The listing builds one solid part. Answer for the finished solid, in the listing's coordinates (mm). A direction names the side the tool comes from. Coordinates: 2 decimals unless noted, no trailing zeros. Order: outer loops, then holes, each group sorted by start corner. A loop starts at its lowest first (then second) coordinate and runs counter-clockwise, first axis right, second up. Notation, with made-up numbers: (-6, -21.5) -> (43, -21.5) arc R16 cw to (43, -14.5) -> close; hole circle Ø11 at (-35, 16). An arc over 180 degrees is marked (long way). Answer in a Markdown table with one row per item. Add a question column.
```python
from build123d import *

# Parameters (mm, degrees)
BOSS_EXTRUDE1_DEPTH     = 2
SKETCH2_W               = 3.5
SKETCH2_H               = 2
CUT_EXTRUDE1_DEPTH      = 22
BOSS_EXTRUDE2_DEPTH     = 7
BOSS_EXTRUDE3_DEPTH     = 6
SKETCH5_R               = 2.25
CUT_EXTRUDE3_DEPTH      = 37
CUT_EXTRUDE3_DEPTH_BACK = 37
FILLET1_R               = 3
FILLET2_R               = 0.5
CUT_EXTRUDE4_DEPTH      = 37
FILLET3_R               = 0.5
FILLET4_R               = 0.5
CUT_EXTRUDE5_DEPTH      = 10
FILLET8_R               = 1
SKETCH8_W               = 0.1
SKETCH8_H               = 1
CUT_EXTRUDE6_DEPTH      = 0.1
SKETCH11_R              = 50.237983701
CUT_EXTRUDE8_DEPTH      = 11
CUT_EXTRUDE8_DEPTH_BACK = 1


with BuildPart() as part:
    # Sketch1 → Boss-Extrude1 (new body)
    with BuildSketch(Plane(origin=(0, 0, 0), x_dir=(1, 0, 0), z_dir=(0, 1, 0))):
        with BuildLine():
            Line((-27.424590139, -24.837307739), (27.424590139, -24.837307739))
            ThreePointArc((27.424590139, -24.837307739), (37, 0), (27.424590139, 24.837307739))
            Line((27.424590139, 24.837307739), (-27.424590139, 24.837307739))
            ThreePointArc((-27.424590139, 24.837307739), (-37, 0), (-27.424590139, -24.837307739))
        make_face()
    extrude(amount=BOSS_EXTRUDE1_DEPTH)

    # Sketch2 → Cut-Extrude1 (cut)
    with BuildSketch(Plane.XZ):
        Polygon((-8, 0), (-8, 9.5), (-11, 9.5), (-11, -9.5), (-8, -9.5), align=None)
        with Locations((-9.75, 0)):
            Rectangle(SKETCH2_W, SKETCH2_H)
    extrude(amount=-CUT_EXTRUDE1_DEPTH, mode=Mode.SUBTRACT)

    # Sketch3 → Boss-Extrude2 (add)
    with BuildSketch(Plane(origin=(0, 2, 0), x_dir=(1, 0, 0), z_dir=(0, 1, 0))):
        Polygon((2.9, 11.6), (2.9, 10.1), (19, 10.1), (20.5, 10.1), (20.5, 11.6), align=None)
        Polygon((20.5, 10.1), (19, 10.1), (19, -10.1), (19, -11.6), (20.5, -11.6), align=None)
        Polygon((19, -11.6), (19, -10.1), (-14.6, -10.1), (-16.1, -10.1), (-16.1, -11.6), align=None)
        Polygon((-14.6, 10.1), (2.9, 10.1), (2.9, 11.6), (-16.1, 11.6), (-16.1, 10.1), align=None)
    extrude(amount=BOSS_EXTRUDE2_DEPTH)

    # Sketch4 → Boss-Extrude3 (add)
    with BuildSketch(Plane.XZ):
        Polygon((-8, 0), (-8.02303658, 9.318964787), (-3, 9.318964787), (-3, -9.5), (-8, -9.5), align=None)
    extrude(amount=BOSS_EXTRUDE3_DEPTH)

    # Sketch5 → Cut-Extrude3 (cut, two sides)
    with BuildSketch(Plane.ZY.offset(8)) as cut_extrude3_sk:
        with Locations((-5.031035213, -2.35)):
            Circle(SKETCH5_R)
        with Locations((5.031035213, -2.35)):
            Circle(SKETCH5_R)
    extrude(amount=CUT_EXTRUDE3_DEPTH, mode=Mode.SUBTRACT)
    extrude(cut_extrude3_sk.sketch, amount=-CUT_EXTRUDE3_DEPTH_BACK, mode=Mode.SUBTRACT)

    # Fillet1
    fillet1_edges = [part.edges().sort_by_distance(p)[0] for p in [
        (-5.5, -6, -9.5),
        (-5.51151829, -6, 9.318964787),
    ]]
    fillet(fillet1_edges, radius=FILLET1_R)

    # Fillet2
    fillet2_edges = [part.edges().sort_by_distance(p)[0] for p in [
        (-37, 2, 0),
        (37, 2, 0),
    ]]
    fillet(fillet2_edges, radius=FILLET2_R)

    # Sketch6 → Cut-Extrude4 (cut)
    with BuildSketch(Plane.XZ):
        with BuildLine():
            Line((-34.696885188, 1.668964787), (-31.296885188, 1.668964787))
            ThreePointArc((-31.296885188, 1.668964787), (-29.596885188, -0.031035213), (-31.296885188, -1.731035213))
            Line((-31.296885188, -1.731035213), (-34.696885188, -1.731035213))
            ThreePointArc((-34.696885188, -1.731035213), (-36.396885188, -0.031035213), (-34.696885188, 1.668964787))
        make_face()
        with BuildLine():
            Line((31.302827177, 1.806746588), (34.702827177, 1.806746588))
            ThreePointArc((34.702827177, 1.806746588), (36.402827177, 0.106746588), (34.702827177, -1.593253412))
            Line((34.702827177, -1.593253412), (31.302827177, -1.593253412))
            ThreePointArc((31.302827177, -1.593253412), (29.602827177, 0.106746588), (31.302827177, 1.806746588))
        make_face()
    extrude(amount=-CUT_EXTRUDE4_DEPTH, mode=Mode.SUBTRACT)

    # Fillet3
    fillet3_edges = [part.edges().sort_by_distance(p)[0] for p in [
        (20.5, 9, 0),
        (2.2, 9, -11.6),
        (2.2, 9, 11.6),
        (1.45, 9, -10.1),
        (19, 9, 0),
        (1.45, 9, 10.1),
    ]]
    fillet(fillet3_edges, radius=FILLET3_R)

    # Fillet4
    fillet4_edges = [part.edges().sort_by_distance(p)[0] for p in [
        (-16.1, 9, -10.85),
        (-16.1, 9, 10.85),
        (-16.1, 5.25, -10.1),
        (-16.1, 5.25, -11.6),
        (-16.1, 8.853553391, -11.453553391),
        (-16.1, 8.853553391, -10.246446609),
        (-16.1, 5.25, 11.6),
        (-16.1, 5.25, 10.1),
        (-16.1, 8.853553391, 10.246446609),
        (-16.1, 8.853553391, 11.453553391),
    ]]
    fillet(fillet4_edges, radius=FILLET4_R)

    # Sketch7 → Cut-Extrude5 (cut)
    with BuildSketch(Plane.XZ):
        Polygon((-19.996885188, 19.968964787), (-10.996885188, 19.968964787), (-10.996885188, 11.968964787), (-28.996885188, 11.968964787), (-28.996885188, 19.968964787), align=None)
        Polygon((11.003114812, 11.968964787), (20.003114812, 11.968964787), (20.003114812, 14.968964787), (20.003114812, 19.968964787), (11.003114812, 19.968964787), align=None)
        Polygon((20.003114812, 14.968964787), (20.003114812, 11.968964787), (29.003114812, 11.968964787), (29.003114812, 19.968964787), (20.003114812, 19.968964787), align=None)
        Polygon((-28.996885188, -12.031035213), (-28.996885188, -20.031035213), (-19.996885188, -20.031035213), (-10.996885188, -20.031035213), (-10.996885188, -12.031035213), align=None)
        Polygon((20.003114812, -20.031035213), (11.003114812, -20.031035213), (11.003114812, -12.031035213), (29.003114812, -12.031035213), (29.003114812, -20.031035213), align=None)
    extrude(amount=-CUT_EXTRUDE5_DEPTH, mode=Mode.SUBTRACT)

    # Fillet8
    fillet8_edges = [part.edges().sort_by_distance(p)[0] for p in [
        (11.003114812, 0, 15.968964787),
        (20.003114812, 0, 11.968964787),
        (29.003114812, 0, 15.968964787),
        (20.003114812, 0, 19.968964787),
        (-28.996885188, 0, -16.031035213),
        (-19.996885188, 0, -20.031035213),
        (-10.996885188, 0, -16.031035213),
        (-19.996885188, 0, -12.031035213),
        (20.003114812, 0, -20.031035213),
        (11.003114812, 0, -16.031035213),
        (20.003114812, 0, -12.031035213),
        (29.003114812, 0, -16.031035213),
        (-19.996885188, 0, 19.968964787),
        (-10.996885188, 0, 15.968964787),
        (-19.996885188, 0, 11.968964787),
        (-28.996885188, 0, 15.968964787),
    ]]
    fillet(fillet8_edges, radius=FILLET8_R)

    # Sketch8 → Cut-Extrude6 (cut)
    with BuildSketch(Plane.XY.offset(24.837307739)):
        with Locations((-0.05, 0.5)):
            Rectangle(SKETCH8_W, SKETCH8_H)
        with Locations((0.05, 0.5)):
            Rectangle(SKETCH8_W, SKETCH8_H)
    extrude(amount=-CUT_EXTRUDE6_DEPTH, mode=Mode.SUBTRACT)

    # Sketch11 → Cut-Extrude8 (cut, two sides)
    with BuildSketch(Plane(origin=(0, 2, 0), x_dir=(1, 0, 0), z_dir=(0, 1, 0))) as cut_extrude8_sk:
        Circle(SKETCH11_R)
    extrude(amount=CUT_EXTRUDE8_DEPTH, mode=Mode.SUBTRACT)
    extrude(cut_extrude8_sk.sketch, amount=-CUT_EXTRUDE8_DEPTH_BACK, mode=Mode.SUBTRACT)


solid = part.part
```
Q1. A cutting plane is placed at A-A (x = 24). Determine the outline of the cut face in (y, z).
Q2. A cutting plane is placed at B-B (z = -15). Determine the outline of the cut face in (x, y).
Q3. Determine the mould class of faces 4 (the face through (-5.54, -2.25, -7.28)), 5 (the face through (-6, -1, 9.319)), 6 (the face through (-3, -3, 0)), 7 (the face through (29.603, 0.493, 0.069)) for opening direction Z: +Z half, -Z half, draft (parallel to the pull), parting line (faces both ways), or undercut.
Q4. A cutting plane is placed at D-D (x = 5). Determine the outline of the cut face in (y, z), then the cut area to 3 significant figures.
Q5. For faces 1 (the face through (-29.597, 0.493, 0.006)), 2 (the face through (-5, -1, -9.5)), 3 (the face through (-37, 0.49, -0.38)), determine the directions among +Z, -Z, +X, -X, +Y, -Y from which every point of the face is accessible in a straight line to the end or side of a thin tool.
Q6. Given pin 1 (4 mm diameter, centred on x = 8.5, y = -3.5, fed in from +Z); pin 2 (1.5 mm diameter, centred on y = -5, z = -2, fed in from +X); pin 3 (0.5 mm diameter, centred on x = -32.5, y = 0.5, fed in from -Z); pin 4 (3.5 mm diameter, centred on x = -6, y = -2, fed in from -Z), each flat-ended and moving along its own axis, determine where each tip first touches the part or whether it passes through.
Q7. A cutting plane is placed at C-C (y = -1.5). Determine the outline of the cut face in (x, z), then the cut area to 3 significant figures.
Q8. Straight lines are drawn through the part: line 1 (Z direction, x = -15, y = 0.75); line 2 (Y direction, x = -12, z = 6.5); line 3 (X direction, y = -0.75, z = -2.5). For each, find the intervals that lie inside material, in ascending order.
Returned:
| question | item | result |
|---|---|---|
| 1 | outline | (0, -24.84) -> (1, -24.84) -> (1, -20.03) arc R1 ccw to (0, -21.03) -> close; (0, -11.03) arc R1 ccw to (1, -12.03) -> (1, 11.97) arc R1 ccw to (0, 10.97) -> close; (0, 20.97) arc R1 ccw to (1, 19.97) -> (1, 24.84) -> (0, 24.84) -> close |
| 2 | outline | (-33.82, 0) -> (-30, 0) arc R1 ccw to (-29, 1) -> (-33.82, 1) -> close; (-11, 1) arc R1 ccw to (-10, 0) -> (10, 0) arc R1 ccw to (11, 1) -> close; (29, 1) arc R1 ccw to (30, 0) -> (33.82, 0) -> (33.82, 1) -> close |
| 3 | face 4 | undercut |
| 3 | face 5 | +Z half |
| 3 | face 6 | draft |
| 3 | face 7 | undercut |
| 4 | outline | (0, -24.84) -> (1, -24.84) -> (1, 24.84) -> (0, 24.84) -> close |
| 4 | area | 49.7 mm² |
| 5 | face 1 | +Y, -Y |
| 5 | face 2 | -Z, +X, -X, -Y |
| 5 | face 3 | -X, +Y, -Y |
| 6 | pin 1 | passes through |
| 6 | pin 2 | stops at x = -3 |
| 6 | pin 3 | stops at z = -18.14 |
| 6 | pin 4 | stops at z = -9.5 |
| 7 | outline | (-8.02, 7.11) -> (-3, 7.11) -> (-3, 9.32) -> (-8.02, 9.32) -> close; (-8.01, 2.95) -> (-8, 0) -> (-8, -2.95) -> (-3, -2.95) -> (-3, 2.95) -> close; (-8, -9.5) -> (-3, -9.5) -> (-3, -7.11) -> (-8, -7.11) -> close |
| 7 | area | 52.5 mm² |
| 8 | line 1 | z = -24.84 to -20.06, -12 to 11.94, 20 to 24.84 |
| 8 | line 2 | y = 0 to 1 |
| 8 | line 3 | x = -8 to -3 |
